```python
from build123d import *

# Parameters (mm, degrees)
CROQUIS1_R              = 15.9
CROQUIS1_R_2            = 13.9
SALIENTE_EXTRUIR1_DEPTH = 22
CROQUIS2_W              = 7
CROQUIS2_H              = 20
CORTAR_EXTRUIR1_DEPTH   = 22


with BuildPart() as part:
    # Croquis1 → Saliente-Extruir1 (new body)
    with BuildSketch(Plane(origin=(0, 0, 0), x_dir=(1, 0, 0), z_dir=(0, 1, 0))):
        Circle(CROQUIS1_R)
        Circle(CROQUIS1_R_2, mode=Mode.SUBTRACT)
    extrude(amount=SALIENTE_EXTRUIR1_DEPTH)

    # Croquis2 → Cortar-Extruir1 (cut)
    with BuildSketch(Plane.XY):
        Rectangle(CROQUIS2_W, CROQUIS2_H)
    extrude(amount=-CORTAR_EXTRUIR1_DEPTH, mode=Mode.SUBTRACT)


solid = part.part
```
The listing builds one solid part. Answer for the finished solid, in the listing's coordinates (mm). A direction names the side the tool comes from. Round coordinates to 2 decimals unless told otherwise and drop trailing zeros. Write each loop counter-clockwise with the first axis right and the second up, starting at its lowest first coordinate (ties: lowest second). Pieces come first, ordered by that corner, then holes. Notation, with made-up numbers: (60.25, -4.5) -> (112.25, -4.5) arc R11 ccw to (112.25, 2.5) -> close; hole circle Ø11 at (-10, 29.25). An arc over 180 degrees is marked (long way). Use CSV: the item, a comma, the result in double quotes. Start each with the question number.
(1) The mould has two halves that part along Z. Classify faces 1 (the face through (-3.45, 10.85, 15.52)), 2 (the face through (-3.01, 10.85, 13.57)), 3 (the face through (-0.1, 0, 14.1)): released by +Z, released by -Z, zero draft, split by the parting line, or undercut.
(2) Section B-B on z = 0 is taken. Give the vertices of the cut face in (x, y).
(3) Section C-C on y = 2 is taken. Give the vertices of the cut face in (x, z).
(4) Each of these flat-tipped pins is pushed along its axis until it touches: pin 1 (2 mm diameter, centred on y = 4.5, z = -4, fed in from -X); pin 2 (2 mm diameter, centred on x = 7, y = 4.5, fed in from -Z); pin 3 (10 mm diameter, centred on x = 7.5, z = 4, fed in from +Y); pin 4 (0.7 mm diameter, centred on x = -0.5, z = -15, fed in from -Y). Where does it stop, or does it pass through?
(5) Consider L1, parallel to Z at x = 0, y = 12.5; L2, parallel to Z at x = -4.5, y = 14.75. Determine where each line is inside the solid, lowest interval first. Write a range as from..to.
(6) Which of the six approach directions +Z, -Z, +X, -X, +Y, -Y give full straight-line access (tool end or side, diameter ignored) to faces 4 (the face through (-0.1, 22, 14.1)), 5 (the face through (0, 10, -15))?
(7) Section A-A on x = 0 is taken. Give the vertices of the cut face in (y, z).
(8) Section D-D on y = 16.5 is taken. Give the vertices of the cut face in (x, z).
A:
1,face 1,"split by the parting line"
1,face 2,"undercut"
1,face 3,"zero draft"
2,outline,"(-15.9, 0) -> (-13.9, 0) -> (-13.9, 22) -> (-15.9, 22) -> close; (13.9, 0) -> (15.9, 0) -> (15.9, 22) -> (13.9, 22) -> close"
3,outline,"(-3.5, -15.51) -> (-3.5, -13.45) arc R13.9 cw (long way) to (3.5, -13.45) -> (3.5, -15.51) arc R15.9 ccw (long way) to start"
4,pin 1,"stops at x = -15.61"
4,pin 2,"stops at z = -14.72"
4,pin 3,"passes through"
4,pin 4,"stops at y = 10"
5,L1,"z = -15.9..-13.9, 13.9..15.9"
5,L2,"z = -15.25..-13.15, 13.15..15.25"
6,face 4,"+Z, -Z, +X, -X, +Y"
6,face 5,"-Z, -Y"
7,outline,"(0, 13.9) -> (22, 13.9) -> (22, 15.9) -> (0, 15.9) -> close; (10, -15.9) -> (22, -15.9) -> (22, -13.9) -> (10, -13.9) -> close"
8,outline,"circle Ø31.8 at (0, 0); hole circle Ø27.8 at (0, 0)"
